Source: CAD feature listing. Evaluate the final solid. Frame: model axes, mm. A direction names the side the tool comes from. Round coordinates to 2 decimals unless told otherwise and drop trailing zeros. Order: outer loops, then holes, each group sorted by start corner. A loop starts at its lowest first (then second) coordinate and runs counter-clockwise, first axis right, second up. Notation, with made-up numbers: M 81.5,47.25 L 117.5,47.25 A16 ccw 117.5,76.25 Z; hole C 24.5,-36 d9. An arc over 180 degrees is marked long. Use one line per item in the form item = value. Start each with the question number.
Q1. Pull-direction query (X, two-part tool) for faces 1 (the flat face through (15.21, 5, 13)), 2 (the flat face through (2, 10, 0)), 3 (the flat face through (21.21, 8, 13)); classes: pulls with the +X half, pulls with the -X half, needs draft (parallel to the pull), parting line crosses it, or undercut.
Q2. Contact query for flat-ended pins moving along their axis: pin 1 (2 mm diameter, centred on x = -12, z = 21, fed in from +Y) (3 decimals); pin 2 (6 mm diameter, centred on y = 27, z = 18.5, fed in from +X); pin 3 (10 mm diameter, centred on y = 27, z = 8, fed in from +X). Output: stop coordinate, or through.
Q3. Section C-C (y = 28.5). Return the cut outline in (x, z).
Q4. Section A-A (z = 12.7). Return the cut outline in (x, y) (3 decimals).
Q5. Reachability of faces 4 (the flat face through (-13, 0, 13)), 5 (the flat face through (11.1, 15.875, 18.2)), 6 (the flat face through (2, 9, 13)) from +Z, -Z, +X, -X, +Y, -Y: full face, straight path, thin tool, end or side. Return the list, or none.
Q6. Section B-B (x = 13.5). Return the cut outline in (y, z) (3 decimals), plus the area to 3 significant figures.
Q7. Section D-D (y = 20). Return the cut outline in (x, z), plus the area to 3 significant figures.
Q8. Material intervals for probe 1 along X at (y, z) = (5.5, 9.25); probe 2 along Y at (x, z) = (1, 8.25) (3 decimals); probe 3 along Y at (x, z) = (-14, 2.25) (3 decimals), sorted ascending.
from build123d import *

# Parameters (mm, degrees)
BOSS_EXTRUDE1_DEPTH = 25.4
SKETCH2_R           = 5
BOSS_EXTRUDE2_DEPTH = 14.5
FILLET1_R           = 5


with BuildPart() as part:
    # Sketch1 → Boss-Extrude1 (new body)
    with BuildSketch(Plane.XY):
        Polygon((-10.189534884, 0), (-10.189534884, 9), (15.210465116, 9), (15.210465116, 0), (21.210465116, 0), (21.210465116, 15.875), (-16.189534884, 15.875), (-16.189534884, 0), align=None)
    extrude(amount=BOSS_EXTRUDE1_DEPTH)

    # Sketch2 → Boss-Extrude2 (add)
    with BuildSketch(Plane(origin=(0, 15.875, 0), x_dir=(1, 0, 0), z_dir=(0, 1, 0))):
        with Locations((2.510465116, -12.7)):
            Circle(SKETCH2_R)
    extrude(amount=BOSS_EXTRUDE2_DEPTH)

    # Fillet1
    fillet1_edges = [part.edges().sort_by_distance(p)[0] for p in [
        (-2.489534884, 15.875, 12.7),
    ]]
    fillet(fillet1_edges, radius=FILLET1_R)


solid = part.part
Results list:
q1.face_1 = undercut
q1.face_2 = needs draft
q1.face_3 = pulls with the +X half
q2.pin_1 = 15.875
q2.pin_2 = 6.65
q2.pin_3 = 7.51
q3.outline = C 2.51,12.7 d10
q4.outline = M -16.19,0 L -10.19,0 L -10.19,9 L 15.21,9 L 15.21,0 L 21.21,0 L 21.21,15.875 L 12.51,15.875 A5 cw 7.51,20.875 L 7.51,30.375 L -2.49,30.375 L -2.49,20.875 A5 cw -7.49,15.875 L -16.19,15.875 Z
q5.face_4 = +Z, -Z, +X, -X, -Y
q5.face_5 = +Y
q5.face_6 = +Z, -Z, -Y
q6.outline = M 9,0 L 15.875,0 L 15.875,25.4 L 9,25.4 Z
q6.area = 175 mm2
q7.outline = C 2.51,12.7 d10.15
q7.area = 81.0 mm2
q8.probe_1 = -16.19 to -10.19, 15.21 to 21.21
q8.probe_2 = 9 to 30.375
q8.probe_3 = 0 to 15.875
